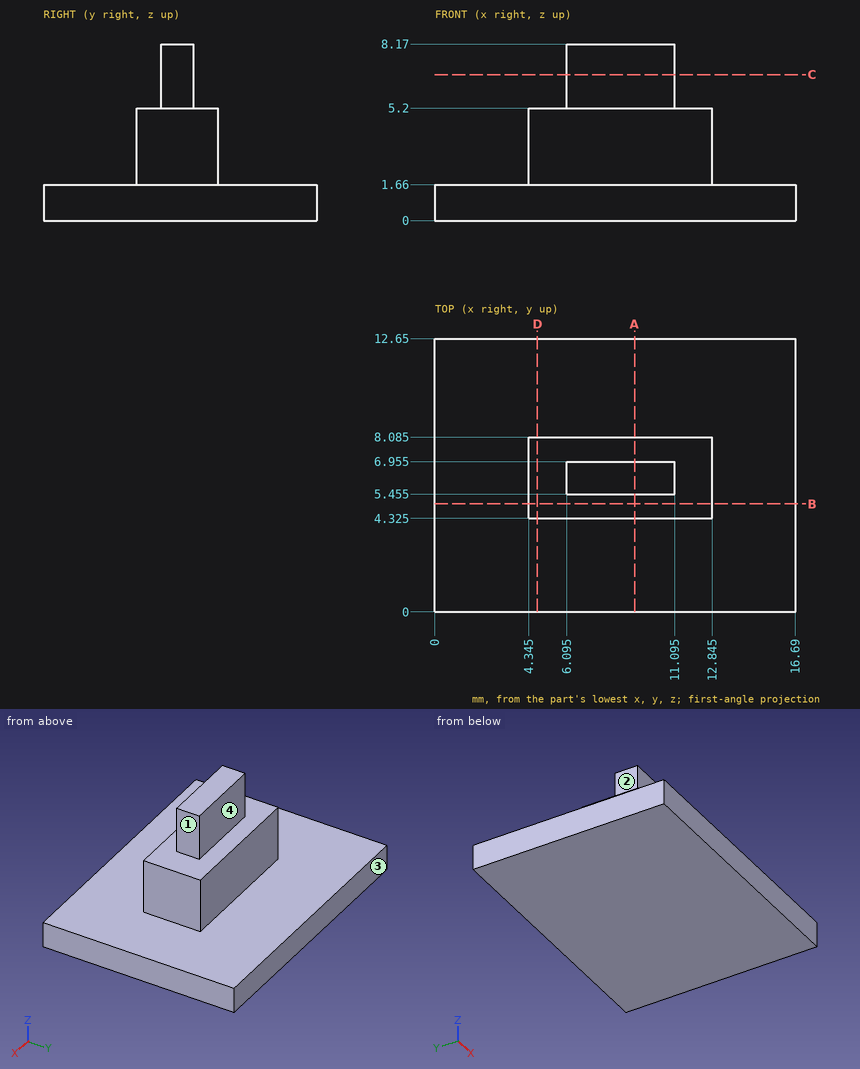
Can you work these out from the drawing? Everything is in mm from the part's minimum corner. A direction names the side the tool comes from. Round coordinates to 2 decimals unless told otherwise and drop trailing zeros. Loops run counter-clockwise (first coordinate to the right, second up) from the corner with the lowest first, then second, coordinate; pieces in that order, holes last. Notation, with made-up numbers: (85, 4.25) - (122, 4.25) arc R6 cw to (122, 15.25) - close; hole circle Ø9 at (47, 60.25). An arc over 180 degrees is marked (long way). Write item = value, one per line. Start each with the question number.
(1) For P1, Ø4, axis at x = 12.5, y = 2, coming from the +Z side; P2, Ø4, axis at x = 4, z = 4.5, coming from the -Y side (3 decimals); P3, Ø1.5, axis at x = 3.5, z = 6, coming from the +Y side; P4, Ø0.8, axis at y = 6.5, z = 6.5, coming from the +X side (3 decimals), each with a flat end and sliding along its axis, tell me the tip position at first contact or that it passes through.
(2) If we section it at A-A (x = 9.25): Please give me the cut outline in (y, z) (3 decimals).
(3) If we section it at D-D (x = 4.75): Please give me the cut outline in (y, z) (3 decimals), and give its area (3 significant figures).
(4) If I drill on probe 1 along Z at (x, y) = (4.5, 7); probe 2 along Z at (x, y) = (12.5, 2.75); probe 3 along X at (y, z) = (7, 2) (3 decimals), over which ranges is the centre line in solid material (lowest first)? Write a range as [from, to].
(5) If we section it at C-C (z = 6.75): Please give me the cut outline in (x, y) (3 decimals).
(6) If we section it at B-B (y = 5): Please give me the cut outline in (x, z) (3 decimals), and give its area (3 significant figures).
(7) For the marked faces 1, 2, 3 and 4, which set-ups out of +Z, -Z, +X, -X, +Y, -Y let a thin tool reach every point of the face, with its end or its side?
Ans:
q1.P1 = 1.66
q1.P2 = 4.325
q1.P3 = through
q1.P4 = 11.095
q2.outline = (0, 0) - (12.65, 0) - (12.65, 1.66) - (8.085, 1.66) - (8.085, 5.2) - (6.955, 5.2) - (6.955, 8.17) - (5.455, 8.17) - (5.455, 5.2) - (4.325, 5.2) - (4.325, 1.66) - (0, 1.66) - close
q3.outline = (0, 0) - (12.65, 0) - (12.65, 1.66) - (8.085, 1.66) - (8.085, 5.2) - (4.325, 5.2) - (4.325, 1.66) - (0, 1.66) - close
q3.area = 34.3 mm²
q4.probe_1 = [0, 5.2]
q4.probe_2 = [0, 1.66]
q4.probe_3 = [4.345, 12.845]
q5.outline = (6.095, 5.455) - (11.095, 5.455) - (11.095, 6.955) - (6.095, 6.955) - close
q6.outline = (0, 0) - (16.69, 0) - (16.69, 1.66) - (12.845, 1.66) - (12.845, 5.2) - (4.345, 5.2) - (4.345, 1.66) - (0, 1.66) - close
q6.area = 57.8 mm²
q7.face_1 = +Z, +X, +Y, -Y
q7.face_2 = +Z, -X, +Y, -Y
q7.face_3 = +Z, -Z, +X, -X, +Y
q7.face_4 = +Z, +X, -X, +Y
